Can you work these out from the model? Positions are in its coordinate system, mm. A direction names the side the tool comes from. Coordinates: 2 decimals unless noted, no trailing zeros. Order: outer loops, then holes, each group sorted by start corner. A loop starts at its lowest first (then second) coordinate and runs counter-clockwise, first axis right, second up. Notation, with made-up numbers: (21, 25.5) -> (38, 25.5) arc R20 ccw to (38, 40.5) -> close; hole circle Ø7 at (83, 52.5). An arc over 180 degrees is marked (long way). Answer as CSV lines item,"result".
from build123d import *

# Parameters (mm, degrees)
SKETCH1_W           = 57
SKETCH1_H           = 37
BOSS_EXTRUDE1_DEPTH = 44
SKETCH2_W           = 38.4
SKETCH2_H           = 36
CUT_EXTRUDE1_DEPTH  = 47
BOSS_EXTRUDE2_DEPTH = 20
BOSS_EXTRUDE3_DEPTH = 20
SKETCH7_W           = 53
SKETCH7_H           = 31
CUT_EXTRUDE4_DEPTH  = 8
SKETCH8_R           = 1.9
CUT_EXTRUDE5_DEPTH  = 40
SKETCH10_W          = 57
SKETCH10_H          = 77
BOSS_EXTRUDE4_DEPTH = 10
SKETCH11_W          = 77
SKETCH11_H          = 8
CUT_EXTRUDE8_DEPTH  = 100


with BuildPart() as part:
    # Sketch1 → Boss-Extrude1 (new body)
    with BuildSketch(Plane(origin=(0, 0, 0), x_dir=(1, 0, 0), z_dir=(0, 1, 0))):
        Rectangle(SKETCH1_W, SKETCH1_H)
    extrude(amount=BOSS_EXTRUDE1_DEPTH)

    # Sketch2 → Cut-Extrude1 (cut)
    with BuildSketch(Plane.XY.offset(18.5)):
        with Locations((0, 18)):
            Rectangle(SKETCH2_W, SKETCH2_H)
    extrude(amount=-CUT_EXTRUDE1_DEPTH, mode=Mode.SUBTRACT)

    # Sketch5 → Boss-Extrude2 (add)
    with BuildSketch(Plane(origin=(0, 0, -18.5), x_dir=(-1, 0, 0), z_dir=(0, 0, -1))):
        Polygon((-19.2, 36), (19.2, 36), (19.2, 0), (28.5, 0), (28.5, 44), (-28.5, 44), (-28.5, 0), (-19.2, 0), align=None)
    extrude(amount=BOSS_EXTRUDE2_DEPTH)

    # Sketch6 → Boss-Extrude3 (add)
    with BuildSketch(Plane.XY.offset(18.5)):
        Polygon((-28.5, 0), (-19.2, 0), (-19.2, 36), (19.2, 36), (19.2, 0), (28.5, 0), (28.5, 44), (-28.5, 44), align=None)
    extrude(amount=BOSS_EXTRUDE3_DEPTH)

    # Sketch7 → Cut-Extrude4 (cut)
    with BuildSketch(Plane(origin=(0, 44, 0), x_dir=(1, 0, 0), z_dir=(0, 1, 0))):
        with Locations((-2, 0)):
            Rectangle(SKETCH7_W, SKETCH7_H)
    extrude(amount=-CUT_EXTRUDE4_DEPTH, mode=Mode.SUBTRACT)

    # Sketch8 → Cut-Extrude5 (cut)
    with BuildSketch(Plane(origin=(0, 44, 0), x_dir=(1, 0, 0), z_dir=(0, 1, 0))):
        with Locations(Location((23.85, -27, 0), (0, 0, 270))):
            Circle(SKETCH8_R)
        with Locations(Location((-23.85, -27, 0), (0, 0, 270))):
            Circle(SKETCH8_R)
        with Locations(Location((-23.85, 27, 0), (0, 0, 270))):
            Circle(SKETCH8_R)
        with Locations(Location((23.85, 27, 0), (0, 0, 270))):
            Circle(SKETCH8_R)
    extrude(amount=-CUT_EXTRUDE5_DEPTH, mode=Mode.SUBTRACT)

    # Sketch10 → Boss-Extrude4 (add)
    with BuildSketch(Plane.XZ):
        Rectangle(SKETCH10_W, SKETCH10_H)
    extrude(amount=BOSS_EXTRUDE4_DEPTH)

    # Sketch11 → Cut-Extrude8 (cut)
    with BuildSketch(Plane.ZY.offset(28.5)):
        with Locations((0, 40)):
            Rectangle(SKETCH11_W, SKETCH11_H)
    extrude(amount=-CUT_EXTRUDE8_DEPTH, mode=Mode.SUBTRACT)


solid = part.part
Q1. If I drill on line 1 (X direction, y = 24, z = -27); line 2 (X direction, y = 28, z = -5); line 3 (Z direction, x = -24, y = 22), over which ranges is the centre line in solid material (lowest first)?
Solution:
line 1,"-28.5 to -25.75, -21.95 to -19.2, 19.2 to 21.95, 25.75 to 28.5"
line 2,"-28.5 to -19.2, 19.2 to 28.5"
line 3,"-38.5 to -28.89, -25.11 to 25.11, 28.89 to 38.5"
Q2. Imagine slicing it at A-A (y = 22). List the corners of the cut face in (x, z) for me, and give its area (3 significant figures).
Solution:
outline,"(-28.5, -38.5) -> (-19.2, -38.5) -> (-19.2, 38.5) -> (-28.5, 38.5) -> close; (19.2, -38.5) -> (28.5, -38.5) -> (28.5, 38.5) -> (19.2, 38.5) -> close; hole circle Ø3.8 at (-23.85, -27); hole circle Ø3.8 at (-23.85, 27); hole circle Ø3.8 at (23.85, -27); hole circle Ø3.8 at (23.85, 27)"
area,"1,390 mm2"
Q3. We'd pull the mould along Z, two halves only. Please class faces 1 (the flat face through (-24, 4, 27)), 2 (the flat face through (-24, 36, -1)), 3 (the flat face through (24, 4, 27)), 4 (the flat face through (-7, -2, 38.5)): pulls with the +Z half, pulls with the -Z half, needs draft (parallel to the pull), parting line crosses it, or undercut.
Solution:
face 1,"undercut"
face 2,"needs draft"
face 3,"undercut"
face 4,"pulls with the +Z half"
Q4. Imagine slicing it at B-B (x = -23.85). List the corners of the cut face in (y, z) for me.
Solution:
outline,"(-10, -38.5) -> (36, -38.5) -> (36, -28.9) -> (4, -28.9) -> (4, -25.1) -> (36, -25.1) -> (36, 25.1) -> (4, 25.1) -> (4, 28.9) -> (36, 28.9) -> (36, 38.5) -> (-10, 38.5) -> close"
Q5. Which directions (+Z, -Z, +X, -X, +Y, -Y) give clear straight access to the entire face, cutting with the end or side of a thin tool? Please do faces 5 (the flat face through (-7, -2, -38.5)), 6 (the cylindrical face through (22.164, 20.224, 27.877)), 7 (the flat face through (19.2, 18, -1)).
Solution:
face 5,"-Z, +X, -X, +Y, -Y"
face 6,"+Y"
face 7,"+Z, -Z, +Y"
Q6. Imagine slicing it at C-C (z = 0). List the corners of the cut face in (x, y) for me, and give its area (3 significant figures).
Solution:
outline,"(-28.5, -10) -> (28.5, -10) -> (28.5, 36) -> (19.2, 36) -> (19.2, 0) -> (-19.2, 0) -> (-19.2, 36) -> (-28.5, 36) -> close"
area,"1,240 mm2"
Q7. For P1, Ø12, axis at x = -4.5, y = 0.5, coming from the -Z side; P2, Ø1.9, axis at x = 24.5, z = -27, coming from the +Y side; P3, Ø19, axis at x = 2, z = 9.5, coming from the +Y side, each with a flat end and sliding along its axis, tell me the tip position at first contact or that it passes through.
Solution:
P1,"z = -38.5"
P2,"y = 4"
P3,"y = 0"
Q8. Imagine slicing it at D-D (z = 27). List the corners of the cut face in (x, y) for me, and give its area (3 significant figures).
Solution:
outline,"(-28.5, -10) -> (28.5, -10) -> (28.5, 36) -> (25.75, 36) -> (25.75, 4) -> (21.95, 4) -> (21.95, 36) -> (19.2, 36) -> (19.2, 0) -> (-19.2, 0) -> (-19.2, 36) -> (-21.95, 36) -> (-21.95, 4) -> (-25.75, 4) -> (-25.75, 36) -> (-28.5, 36) -> close"
area,"996 mm2"
